Input: part model. Units: mm. Frame: model coordinates. Round coordinates to 2 decimals unless told otherwise and drop trailing zeros. Order: outer loops, then holes, each group sorted by start corner. A loop starts at its lowest first (then second) coordinate and runs counter-clockwise, first axis right, second up. Notation, with made-up numbers: (-22.75, -12) -> (11.25, -12) arc R26 ccw to (11.25, 21) -> close; hole circle Ø9 at (41, 20). An arc over 180 degrees is marked (long way). Use a Markdown table: item, result.
from build123d import *

# Parameters (mm, degrees)
SKETCH_1_R      = 11.5
EXTRUDE_1_DEPTH = 16
SKETCH_2_R      = 0.3
EXTRUDE_2_DEPTH = 4
FILLET_1_R      = 1


with BuildPart() as part:
    # 草图1 → 凸台-拉伸1 (new body)
    with BuildSketch(Plane(origin=(0, 0, 0), x_dir=(1, 0, 0), z_dir=(0, 1, 0))):
        with Locations(Location((0, 0, 0), (0, 0, 270))):
            Circle(SKETCH_1_R)
    extrude(amount=EXTRUDE_1_DEPTH)

    # 草图2 → 凸台-拉伸2 (add)
    with BuildSketch(Plane.XZ):
        with Locations(Location((-7.5, 0, 0), (0, 0, 90))):
            Circle(SKETCH_2_R)
        with Locations(Location((7.5, 0, 0), (0, 0, 90))):
            Circle(SKETCH_2_R)
    extrude(amount=EXTRUDE_2_DEPTH)

    # 草图3 → 切除-旋转1 (revolve, cut)
    with BuildSketch(Plane(origin=(0, 19, 0), x_dir=(1, 0, 0), z_dir=(0, 0, -1))):
        Polygon((0, 3), (-2.5, 3), (-2.5, 4.5), (-10, 4.5), (-10, 8), (0, 8), align=None)
    revolve(axis=Axis((0, 34.240243578, 0), (0, -1, 0)), mode=Mode.SUBTRACT)

    # 圆角1
    fillet_1_edges = [part.edges().sort_by_distance(p)[0] for p in [
        (0, 0, -11.5),
        (0, 16, -11.5),
    ]]
    fillet(fillet_1_edges, radius=FILLET_1_R)


solid = part.part
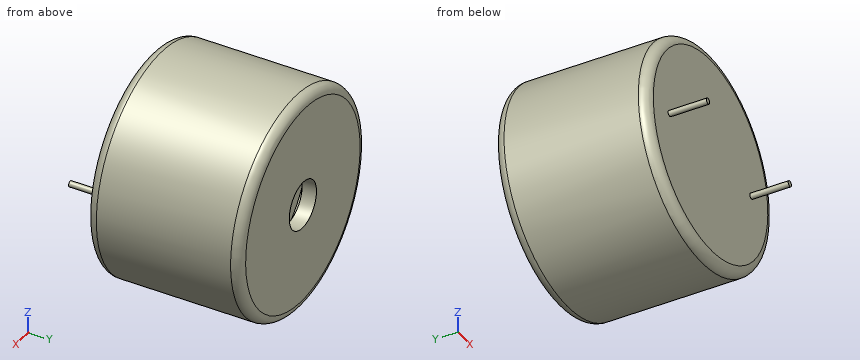
1) Cut plane A-A on x = 0. Return loops of the section in (y, z).
Results found:
| item | result |
|---|---|
| outline | (0, -10.5) arc R1 ccw to (1, -11.5) -> (15, -11.5) arc R1 ccw to (16, -10.5) -> (16, -2.5) -> (14.5, -2.5) -> (14.5, -10) -> (11, -10) -> (11, 10) -> (14.5, 10) -> (14.5, 2.5) -> (16, 2.5) -> (16, 10.5) arc R1 ccw to (15, 11.5) -> (1, 11.5) arc R1 ccw to (0, 10.5) -> close |
2) Cut plane B-B on y = 12. Return loops of the section in (x, z).
Results found:
| item | result |
|---|---|
| outline | circle Ø23 at (0, 0); hole circle Ø20 at (0, 0) |
3) Line query: L1, parallel to X at y = 13, z = 0; L2, parallel to X at y = 14.95, z = 0; L3, parallel to Y at x = -7.25, z = -4.75. Output: solid intervals per line, ascending. Write a range as [from, to].
Results found:
| item | result |
|---|---|
| L1 | x = [-11.5, -10], [10, 11.5] |
| L2 | x = [-11.5, -2.5], [2.5, 11.5] |
| L3 | y = [0, 11], [14.5, 16] |
4) Pin query (flat end, axial travel): pin 1 Ø6 at (y, z) = (1.5, 7) entering from +X; pin 2 Ø5 at (y, z) = (9.5, -3) entering from +X; pin 3 Ø1 at (x, y) = (-5, 9) entering from -Z; pin 4 Ø10 at (x, y) = (3.5, 1) entering from +Z. Return the tip coordinate at first contact, or that it passes through.
Results found:
| item | result |
|---|---|
| pin 1 | stops at x = 10.78 |
| pin 2 | stops at x = 11.49 |
| pin 3 | stops at z = -10.58 |
| pin 4 | stops at z = 11.5 |
5) Cut plane C-C on y = 4.75. Return loops of the section in (x, z).
Results found:
| item | result |
|---|---|
| outline | circle Ø23 at (0, 0) |
6) Cut plane D-D on y = 0.5. Return loops of the section in (x, z), and give its area (3 significant figures).
Results found:
| item | result |
|---|---|
| outline | circle Ø22.73 at (0, 0) |
| area | 406 mm² |
